```python
from build123d import *

# Parameters (mm, degrees)
PAD_DEPTH         = 1.5
CYLINDER001_R     = 2.2
CYLINDER001_DEPTH = 10
CYLINDER_R        = 3.5
CYLINDER_DEPTH    = 10
BOX001_W          = 1.6
BOX001_H          = 14
BOX001_DEPTH      = 20
FILLET001_R       = 3
BOX_W             = 20
BOX_H             = 14
BOX_DEPTH         = 6
FILLET_R          = 2


with BuildPart() as side_wall_body:
    # Sketch → Pad (new body)
    with BuildSketch(Plane.XZ):
        with BuildLine():
            Line((0, 21.297815), (0, 0))
            Line((0, 0), (14.6909, 0))
            add(Edge.make_bspline(
                [(0, 21.297815), (3.272985, 21.659939), (5.756082, 19.125105), (7.618405, 16.072966), (10.515349, 12.71044), (13.308836, 9.192718), (13.722685, 5.778458), (14.6909, 0)],
                knots=[0, 0, 0, 0, 0.2, 0.4, 0.6, 0.8, 1, 1, 1, 1], degree=3))
        make_face()
    extrude(amount=PAD_DEPTH)


with BuildPart() as side_wall_fusion:
    # Part__Mirroring: instance of side wall body
    add(side_wall_body.part.mirror(Plane(origin=(0, 5.5, 0), x_dir=(1, 0, 0), z_dir=(0, 1, 0))))

    # Fusion002: union side wall body
    add(side_wall_body.part)


with BuildPart() as side_wall_fusion_1:
    # Fusion002 placement: moved
    add(side_wall_fusion.part.moved(Location((0, 1.5, 0))))


with BuildPart() as bolt_hole:
    # Cylinder001 → Cylinder001 (new body)
    with BuildSketch(Plane(origin=(15, 7, -4), x_dir=(1, 0, 0), z_dir=(0, 0, 1))):
        Circle(CYLINDER001_R)
    extrude(amount=CYLINDER001_DEPTH)


with BuildPart() as hole_fusion:
    # Cylinder → Cylinder (new body)
    with BuildSketch(Plane(origin=(-3, 7, 20.5), x_dir=(0, 0, -1), z_dir=(1, 0, 0))):
        Circle(CYLINDER_R)
    extrude(amount=CYLINDER_DEPTH)

    # Fusion001: union bolt hole
    add(bolt_hole.part)


with BuildPart() as socket_fillet:
    # Box001 → Box001 (new body)
    with BuildSketch(Plane.XY.offset(6)):
        with Locations((0.8, 7)):
            Rectangle(BOX001_W, BOX001_H)
    extrude(amount=BOX001_DEPTH)

    # Fillet001
    fillet001_edges = [socket_fillet.edges().sort_by_distance(p)[0] for p in [
        (0.8, 0, 26),
        (0.8, 14, 26),
    ]]
    fillet(fillet001_edges, radius=FILLET001_R)


with BuildPart() as audio_socket_fusion:
    # Box → Box (new body)
    with BuildSketch(Plane.XY):
        with Locations((10, 7)):
            Rectangle(BOX_W, BOX_H)
    extrude(amount=BOX_DEPTH)

    # Fillet
    fillet_edges = [audio_socket_fusion.edges().sort_by_distance(p)[0] for p in [
        (20, 0, 3),
        (20, 14, 3),
    ]]
    fillet(fillet_edges, radius=FILLET_R)

    # Fusion: union socket fillet
    add(socket_fillet.part)

    # Cut: cut hole fusion
    add(hole_fusion.part, mode=Mode.SUBTRACT)

    # Fusion003: union side wall fusion
    add(side_wall_fusion_1.part)


solid = audio_socket_fusion.part
```
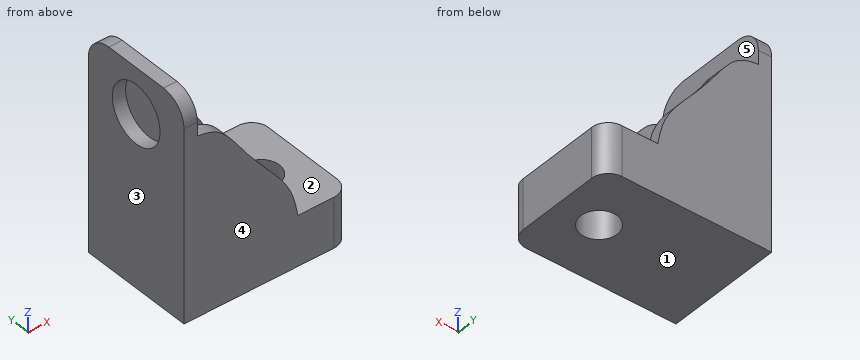
Part model, mm, in its own coordinate system. Face numbers are marked on the shaded views. A direction names the side the tool comes from. Round coordinates to 2 decimals unless told otherwise and drop trailing zeros. Order: outer loops, then holes, each group sorted by start corner. A loop starts at its lowest first (then second) coordinate and runs counter-clockwise, first axis right, second up. Notation, with made-up numbers: M 39.25,11 L 64.25,11 A15 ccw 64.25,36 Z; hole C -22.5,33 d11. An arc over 180 degrees is marked long. Put each result on its own line as item: value. Start each with the question number.
1. Slice it at B-B on z = 4.75. List the corners of the cut face in (x, y), then the cut area to 3 significant figures.
2. Two-plate mould, pull along Y, no slides. Class the marked faces 3, 4 and 5: +Y half, -Y half, draft (parallel to the pull), parting line (faces both ways), or undercut.
3. Drill centre lines: probe 1 along Y at (x, z) = (1.75, 15.5); probe 2 along X at (y, z) = (7, 4.05); probe 3 along Z at (x, y) = (0.4, 7). Where is each one in solid material? Low to high. Write a range as [from, to].
4. Drop flat-ended pins along their axis: pin 1 (2 mm diameter, centred on x = 6, y = 1.5, fed in from +Z); pin 2 (3.5 mm diameter, centred on x = 10.5, z = 16, fed in from +Y); pin 3 (8 mm diameter, centred on y = 7, z = 20.5, fed in from +X). Give the stop position or say it passes through.
5. Slice it at C-C on y = 4. List the corners of the cut face in (x, z).
6. Tool access for the marked faces 1 and 2: list every direction of +Z, -Z, +X, -X, +Y, -Y with a clear straight run to the whole face (end or side of a thin tool).
7. Slice it at A-A on x = 15. List the corners of the cut face in (y, z), then the cut area to 3 significant figures.
8. Slice it at D-D on z = 23.5. List the corners of the cut face in (x, y).
Findings:
1. outline: M 0,0 L 18,0 A2 ccw 20,2 L 20,12 A2 ccw 18,14 L 0,14 Z; hole C 15,7 d4.4
1. area: 263 mm2
2. face 3: draft
2. face 4: -Y half
2. face 5: undercut
3. probe 1: [0, 1.5], [12.5, 14]
3. probe 2: [0, 12.8], [17.2, 20]
3. probe 3: [0, 17], [24, 26]
4. pin 1: z = 19.77
4. pin 2: through
4. pin 3: x = 1.6
5. outline: M 0,0 L 20,0 L 20,6 L 1.6,6 L 1.6,18.7 L 0,18.7 Z; M 0,22.3 L 1.6,22.3 L 1.6,26 L 0,26 Z
6. face 1: -Z, +X, -X, +Y, -Y
6. face 2: +Z, +X
7. outline: M 0,0 L 4.8,0 L 4.8,6 L 0,6 Z; M 9.2,0 L 14,0 L 14,6 L 9.2,6 Z
7. area: 57.6 mm2
8. outline: M 0,0.04 L 1.6,0.04 L 1.6,5.2 L 0,5.2 Z; M 0,8.8 L 1.6,8.8 L 1.6,13.96 L 0,13.96 Z
